from build123d import *

# Parameters (mm, degrees)
SKETCH1_R           = 4.7625
BOSS_EXTRUDE1_DEPTH = 55.88
SKETCH2_R           = 3.81
BOSS_EXTRUDE2_DEPTH = 38.1
SKETCH3_W           = 1.27
SKETCH3_H           = 6.35
CUT_EXTRUDE1_DEPTH  = 19.05
SKETCH4_R           = 1.5875
CUT_EXTRUDE2_DEPTH  = 38.1
FILLET2_R           = 3.81
BOSS_EXTRUDE3_START = 45.72
BOSS_EXTRUDE3_DEPTH = 6.35


with BuildPart() as part:
    # Sketch1 → Boss-Extrude1 (new body)
    with BuildSketch(Plane.XY):
        Circle(SKETCH1_R)
    extrude(amount=BOSS_EXTRUDE1_DEPTH)

    # Sketch2 → Boss-Extrude2 (add)
    with BuildSketch(Plane(origin=(0, 0, 0), x_dir=(-1, 0, 0), z_dir=(0, 0, -1))):
        with Locations(Location((0, 0, 0), (0, 0, 180))):
            Circle(SKETCH2_R)
    extrude(amount=BOSS_EXTRUDE2_DEPTH)

    # Sketch3 → Cut-Extrude1 (cut, symmetric)
    with BuildSketch(Plane(origin=(0, 0, 0), x_dir=(1, 0, 0), z_dir=(0, 1, 0))):
        with Locations((-3.175, 3.175)):
            Rectangle(SKETCH3_W, SKETCH3_H)
        with Locations((3.175, 3.175)):
            Rectangle(SKETCH3_W, SKETCH3_H)
    extrude(amount=CUT_EXTRUDE1_DEPTH, both=True, mode=Mode.SUBTRACT)

    # Sketch4 → Cut-Extrude2 (cut)
    with BuildSketch(Plane(origin=(0, 0, -38.1), x_dir=(-1, 0, 0), z_dir=(0, 0, -1))):
        Circle(SKETCH4_R)
    extrude(amount=-CUT_EXTRUDE2_DEPTH, mode=Mode.SUBTRACT)

    # Fillet2
    fillet2_edges = [part.edges().sort_by_distance(p)[0] for p in [
        (-4.7625, 0, 55.88),
    ]]
    fillet(fillet2_edges, radius=FILLET2_R)

    # Sketch7 → Boss-Extrude3 (add)
    with BuildSketch(Plane.XY.offset(BOSS_EXTRUDE3_START)):
        Polygon((5.701507332, -2.824699621), (5.297015296, 3.525300379), (-0.404492036, 6.35), (-5.701507332, 2.824699621), (-5.297015296, -3.525300379), (0.404492036, -6.35), align=None)
    extrude(amount=BOSS_EXTRUDE3_DEPTH)


solid = part.part
Work out the finished part from the listing and answer in its coordinate system (mm). A direction names the side the tool comes from. Round coordinates to 2 decimals unless told otherwise and drop trailing zeros. Write each loop counter-clockwise with the first axis right and the second up, starting at its lowest first coordinate (ties: lowest second). Pieces come first, ordered by that corner, then holes. Notation, with made-up numbers: (52.25, 1.5) -> (103.25, 1.5) arc R29 cw to (103.25, 30.5) -> close; hole circle Ø11 at (55, 33.5). An arc over 180 degrees is marked (long way). Answer as CSV lines item,"result". Start each with the question number.
(1) The mould has two halves that part along X. Classify faces 4 (the flat face through (5.5, 0.31, 48.85)), 5 (the cylindrical face through (0.34, -1.55, -19.32)), 6 (the flat face through (-5.5, -0.31, 48.85)): +X half, -X half, draft (parallel to the pull), parting line (faces both ways), or undercut.
(2) Find the intervals of material crossed by probe 1 along Y at (x, z) = (0, -27); probe 2 along X at (y, z) = (-0.25, -28); probe 3 along Z at (x, y) = (-3.25, 1.5), in increasing order.
(3) A tool of negligible diameter and unlimited length cuts with its end or side. For faces 1 (the flat face through (-2.54, 0, -3)), 2 (the flat face through (2.54, 0, -3)), 3 (the cylindrical face through (-3.78, -2.9, 22.54)), from which of +Z, -Z, +X, -X, +Y, -Y can it reach the whole face along a straight path? Write none if from no direction.
(4) Each of these flat-tipped pins is pushed along its axis until it touches: pin 1 (4.5 mm diameter, centred on y = 1, z = -3, fed in from -X); pin 2 (4 mm diameter, centred on y = 4, z = 5, fed in from +X); pin 3 (1.7 mm diameter, centred on y = 1, z = -4.5, fed in from +X). Where does it stop, or does it pass through?
(5) The part is cut by section B-B, the plane z = 43.5. Give the vertices of the cut face in (x, y) (1 decimal), then the cut area to 3 significant figures.
(6) The part is cut by section A-A, the plane z = -24.5. Give the vertices of the cut face in (x, y) (1 decimal).
Output values:
1,face 4,"+X half"
1,face 5,"undercut"
1,face 6,"-X half"
2,probe 1,"y = -3.81 to -1.59, 1.59 to 3.81"
2,probe 2,"x = -3.8 to -1.57, 1.57 to 3.8"
2,probe 3,"z = -38.1 to -6.35, 0 to 54.83"
3,face 1,"-X, +Y, -Y"
3,face 2,"+X, +Y, -Y"
3,face 3,"-Z"
4,pin 1,"stops at x = -2.54"
4,pin 2,"stops at x = 4.32"
4,pin 3,"stops at x = 2.54"
5,outline,"circle Ø9.5 at (0, 0)"
5,area,"71.3 mm²"
6,outline,"circle Ø7.6 at (0, 0); hole circle Ø3.2 at (0, 0)"
